Part model, mm, in its own coordinate system. Give positions to 0.01 mm unless a question says otherwise; leave off trailing zeros. Write each loop counter-clockwise with the first axis right and the second up, starting at its lowest first coordinate (ties: lowest second). Pieces come first, ordered by that corner, then holes. Notation, with made-up numbers: M 55,14 L 75,14 A16 ccw 75,33 Z; hole C 79.5,88.5 d3. An arc over 180 degrees is marked long. Use CSV: the item, a comma, the result in double quotes. Start each with the question number.
1. Band-saw the part on D-D, the plane x = 22.5. List the corners of the cut face in (y, z).
2. Drill centre lines: line 1 along X through (y, z) = (2.5, 0); line 2 along Z through (x, y) = (1, 2.4); line 3 along X through (y, z) = (1.2, -1). Where is each one in solid material? Low to high. Write a range as from..to.
3. Drop flat-ended pins along their axis: pin 1 Ø1 at (x, y) = (12, 2.5) entering from -Z; pin 2 Ø1 at (x, y) = (-5, 1.5) entering from -Z. Give the stop position or say it passes through.
4. Band-saw the part on A-A, the plane z = -81. List the corners of the cut face in (x, y), then the cut area to 3 significant figures.
5. Band-saw the part on B-B, the plane y = 2.05. Count the separate pieces of the cut face and the enclosed holes in it, then the cut area to 3 significant figures.
6. Band-saw the part on C-C, the plane z = -70. List the corners of the cut face in (x, y), then the cut area to 3 significant figures.
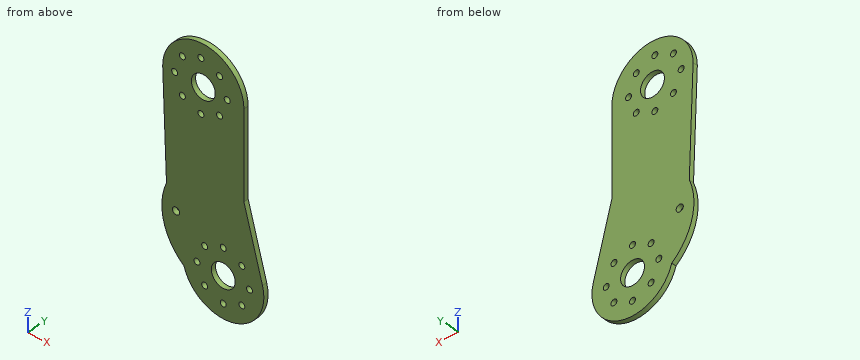
from build123d import *

# Parameters (mm, degrees)
RESSALTO_EXTRUS_O1_DEPTH      = 3
CORTE_EXTRUS_O8_REACH         = 92.666
ESBO_O7_R                     = 1.25
CORTE_EXTRUS_O9_REACH         = 92.666
ESBO_O8_R                     = 5
ESBO_O8_R_2                   = 1.5
CORTE_EXTRUS_O11_REACH        = 92.666
ESBO_O9_R                     = 1.25
CORTE_EXTRUS_O12_REACH        = 92.666
ESBO_O11_R                    = 5
CONVERTER_S_LIDO1_OUTLINE_R   = 1.25
CONVERTER_S_LIDO1_OUTLINE_R_2 = 5
CONVERTER_S_LIDO1_OUTLINE_R_3 = 1.5
CONVERTER_S_LIDO1_DEPTH       = 1


# Read off the part's stored shape, not the designer's step: Converter-Sólido1
with BuildPart() as part:
    # Esboço1 → Ressalto-extrusão1 (new body)
    with BuildSketch(Plane(origin=(0, 0, 0), x_dir=(1, 0, 0), z_dir=(0, 1, 0))):
        with BuildLine():
            Line((17, 36.622301445), (24.764571353, 65.600076233))
            ThreePointArc((24.764571353, 65.600076233), (12.765450327, 86.414910724), (-8.065221434, 74.443304555))
            ThreePointArc((-8.065221434, 74.443304555), (-16.588225274, 61.125706966), (-15.416069793, 45.357826591))
            Line((-15.416069793, 45.357826591), (-17, 0))
            ThreePointArc((-17, 0), (0, -17), (17, 0))
            Line((17, 0), (17, 36.622301445))
        make_face()
    extrude(amount=RESSALTO_EXTRUS_O1_DEPTH)

    # Esboço7 → Corte-extrusão8 (cut, up to next)
    with BuildSketch(Plane.XZ, mode=Mode.PRIVATE) as corte_extrus_o8_sk1:
        with Locations(Location((-1, -11, 0), (0, 0, 270))):
            Circle(ESBO_O7_R)
    corte_extrus_o8_tool1 = extrude(corte_extrus_o8_sk1.sketch, amount=-CORTE_EXTRUS_O8_REACH, mode=Mode.PRIVATE) & part.part
    # Esboço7 → Corte-extrusão8 (cut, up to next)
    with BuildSketch(Plane.XZ, mode=Mode.PRIVATE) as corte_extrus_o8_sk2:
        with Locations(Location((-8.778174593, -7.778174593, 0), (0, 0, 270))):
            Circle(ESBO_O7_R)
    corte_extrus_o8_tool2 = extrude(corte_extrus_o8_sk2.sketch, amount=-CORTE_EXTRUS_O8_REACH, mode=Mode.PRIVATE) & part.part
    # Esboço7 → Corte-extrusão8 (cut, up to next)
    with BuildSketch(Plane.XZ, mode=Mode.PRIVATE) as corte_extrus_o8_sk3:
        with Locations(Location((-12, 0, 0), (0, 0, 270))):
            Circle(ESBO_O7_R)
    corte_extrus_o8_tool3 = extrude(corte_extrus_o8_sk3.sketch, amount=-CORTE_EXTRUS_O8_REACH, mode=Mode.PRIVATE) & part.part
    # Esboço7 → Corte-extrusão8 (cut, up to next)
    with BuildSketch(Plane.XZ, mode=Mode.PRIVATE) as corte_extrus_o8_sk4:
        with Locations(Location((-8.778174593, 7.778174593, 0), (0, 0, 270))):
            Circle(ESBO_O7_R)
    corte_extrus_o8_tool4 = extrude(corte_extrus_o8_sk4.sketch, amount=-CORTE_EXTRUS_O8_REACH, mode=Mode.PRIVATE) & part.part
    # Esboço7 → Corte-extrusão8 (cut, up to next)
    with BuildSketch(Plane.XZ, mode=Mode.PRIVATE) as corte_extrus_o8_sk5:
        with Locations(Location((-1, 11, 0), (0, 0, 270))):
            Circle(ESBO_O7_R)
    corte_extrus_o8_tool5 = extrude(corte_extrus_o8_sk5.sketch, amount=-CORTE_EXTRUS_O8_REACH, mode=Mode.PRIVATE) & part.part
    # Esboço7 → Corte-extrusão8 (cut, up to next)
    with BuildSketch(Plane.XZ, mode=Mode.PRIVATE) as corte_extrus_o8_sk6:
        with Locations(Location((6.778174593, 7.778174593, 0), (0, 0, 270))):
            Circle(ESBO_O7_R)
    corte_extrus_o8_tool6 = extrude(corte_extrus_o8_sk6.sketch, amount=-CORTE_EXTRUS_O8_REACH, mode=Mode.PRIVATE) & part.part
    # Esboço7 → Corte-extrusão8 (cut, up to next)
    with BuildSketch(Plane.XZ, mode=Mode.PRIVATE) as corte_extrus_o8_sk7:
        with Locations(Location((10, 0, 0), (0, 0, 270))):
            Circle(ESBO_O7_R)
    corte_extrus_o8_tool7 = extrude(corte_extrus_o8_sk7.sketch, amount=-CORTE_EXTRUS_O8_REACH, mode=Mode.PRIVATE) & part.part
    # Esboço7 → Corte-extrusão8 (cut, up to next)
    with BuildSketch(Plane.XZ, mode=Mode.PRIVATE) as corte_extrus_o8_sk8:
        with Locations(Location((6.778174593, -7.778174593, 0), (0, 0, 270))):
            Circle(ESBO_O7_R)
    corte_extrus_o8_tool8 = extrude(corte_extrus_o8_sk8.sketch, amount=-CORTE_EXTRUS_O8_REACH, mode=Mode.PRIVATE) & part.part
    add(corte_extrus_o8_tool1.solids().sort_by_distance((-1, 0, -11))[0], mode=Mode.SUBTRACT)
    add(corte_extrus_o8_tool2.solids().sort_by_distance((-8.778175, 0, -7.778175))[0], mode=Mode.SUBTRACT)
    add(corte_extrus_o8_tool3.solids().sort_by_distance((-12, 0, 0))[0], mode=Mode.SUBTRACT)
    add(corte_extrus_o8_tool4.solids().sort_by_distance((-8.778175, 0, 7.778175))[0], mode=Mode.SUBTRACT)
    add(corte_extrus_o8_tool5.solids().sort_by_distance((-1, 0, 11))[0], mode=Mode.SUBTRACT)
    add(corte_extrus_o8_tool6.solids().sort_by_distance((6.778175, 0, 7.778175))[0], mode=Mode.SUBTRACT)
    add(corte_extrus_o8_tool7.solids().sort_by_distance((10, 0, 0))[0], mode=Mode.SUBTRACT)
    add(corte_extrus_o8_tool8.solids().sort_by_distance((6.778175, 0, -7.778175))[0], mode=Mode.SUBTRACT)

    # Esboço8 → Corte-extrusão9 (cut, up to next)
    with BuildSketch(Plane(origin=(0, 3, 0), x_dir=(1, 0, 0), z_dir=(0, 1, 0)), mode=Mode.PRIVATE) as corte_extrus_o9_sk1:
        with Locations(Location((0, 0, 0), (0, 0, 270))):
            Circle(ESBO_O8_R)
    corte_extrus_o9_tool1 = extrude(corte_extrus_o9_sk1.sketch, amount=-CORTE_EXTRUS_O9_REACH, mode=Mode.PRIVATE) & part.part
    # Esboço8 → Corte-extrusão9 (cut, up to next)
    with BuildSketch(Plane(origin=(0, 3, 0), x_dir=(1, 0, 0), z_dir=(0, 1, 0)), mode=Mode.PRIVATE) as corte_extrus_o9_sk2:
        with Locations(Location((-11.416069793, 54.443304555, 0), (0, 0, 270))):
            Circle(ESBO_O8_R_2)
    corte_extrus_o9_tool2 = extrude(corte_extrus_o9_sk2.sketch, amount=-CORTE_EXTRUS_O9_REACH, mode=Mode.PRIVATE) & part.part
    add(corte_extrus_o9_tool1.solids().sort_by_distance((0, 3, 0))[0], mode=Mode.SUBTRACT)
    add(corte_extrus_o9_tool2.solids().sort_by_distance((-11.41607, 3, -54.443305))[0], mode=Mode.SUBTRACT)

    # Esboço9 → Corte-extrusão11 (cut, up to next)
    with BuildSketch(Plane(origin=(0, 3, 0), x_dir=(1, 0, 0), z_dir=(0, 1, 0)), mode=Mode.PRIVATE) as corte_extrus_o11_sk1:
        with Locations(Location((8.343832306, 81, 0), (0, 0, 270))):
            Circle(ESBO_O9_R)
    corte_extrus_o11_tool1 = extrude(corte_extrus_o11_sk1.sketch, amount=-CORTE_EXTRUS_O11_REACH, mode=Mode.PRIVATE) & part.part
    # Esboço9 → Corte-extrusão11 (cut, up to next)
    with BuildSketch(Plane(origin=(0, 3, 0), x_dir=(1, 0, 0), z_dir=(0, 1, 0)), mode=Mode.PRIVATE) as corte_extrus_o11_sk2:
        with Locations(Location((16.122006899, 77.778174593, 0), (0, 0, 270))):
            Circle(ESBO_O9_R)
    corte_extrus_o11_tool2 = extrude(corte_extrus_o11_sk2.sketch, amount=-CORTE_EXTRUS_O11_REACH, mode=Mode.PRIVATE) & part.part
    # Esboço9 → Corte-extrusão11 (cut, up to next)
    with BuildSketch(Plane(origin=(0, 3, 0), x_dir=(1, 0, 0), z_dir=(0, 1, 0)), mode=Mode.PRIVATE) as corte_extrus_o11_sk3:
        with Locations(Location((19.343832306, 70, 0), (0, 0, 270))):
            Circle(ESBO_O9_R)
    corte_extrus_o11_tool3 = extrude(corte_extrus_o11_sk3.sketch, amount=-CORTE_EXTRUS_O11_REACH, mode=Mode.PRIVATE) & part.part
    # Esboço9 → Corte-extrusão11 (cut, up to next)
    with BuildSketch(Plane(origin=(0, 3, 0), x_dir=(1, 0, 0), z_dir=(0, 1, 0)), mode=Mode.PRIVATE) as corte_extrus_o11_sk4:
        with Locations(Location((16.122006899, 62.221825407, 0), (0, 0, 270))):
            Circle(ESBO_O9_R)
    corte_extrus_o11_tool4 = extrude(corte_extrus_o11_sk4.sketch, amount=-CORTE_EXTRUS_O11_REACH, mode=Mode.PRIVATE) & part.part
    # Esboço9 → Corte-extrusão11 (cut, up to next)
    with BuildSketch(Plane(origin=(0, 3, 0), x_dir=(1, 0, 0), z_dir=(0, 1, 0)), mode=Mode.PRIVATE) as corte_extrus_o11_sk5:
        with Locations(Location((8.343832306, 59, 0), (0, 0, 270))):
            Circle(ESBO_O9_R)
    corte_extrus_o11_tool5 = extrude(corte_extrus_o11_sk5.sketch, amount=-CORTE_EXTRUS_O11_REACH, mode=Mode.PRIVATE) & part.part
    # Esboço9 → Corte-extrusão11 (cut, up to next)
    with BuildSketch(Plane(origin=(0, 3, 0), x_dir=(1, 0, 0), z_dir=(0, 1, 0)), mode=Mode.PRIVATE) as corte_extrus_o11_sk6:
        with Locations(Location((0.565657713, 62.221825407, 0), (0, 0, 270))):
            Circle(ESBO_O9_R)
    corte_extrus_o11_tool6 = extrude(corte_extrus_o11_sk6.sketch, amount=-CORTE_EXTRUS_O11_REACH, mode=Mode.PRIVATE) & part.part
    # Esboço9 → Corte-extrusão11 (cut, up to next)
    with BuildSketch(Plane(origin=(0, 3, 0), x_dir=(1, 0, 0), z_dir=(0, 1, 0)), mode=Mode.PRIVATE) as corte_extrus_o11_sk7:
        with Locations(Location((-2.656167694, 70, 0), (0, 0, 270))):
            Circle(ESBO_O9_R)
    corte_extrus_o11_tool7 = extrude(corte_extrus_o11_sk7.sketch, amount=-CORTE_EXTRUS_O11_REACH, mode=Mode.PRIVATE) & part.part
    # Esboço9 → Corte-extrusão11 (cut, up to next)
    with BuildSketch(Plane(origin=(0, 3, 0), x_dir=(1, 0, 0), z_dir=(0, 1, 0)), mode=Mode.PRIVATE) as corte_extrus_o11_sk8:
        with Locations(Location((0.565657713, 77.778174593, 0), (0, 0, 270))):
            Circle(ESBO_O9_R)
    corte_extrus_o11_tool8 = extrude(corte_extrus_o11_sk8.sketch, amount=-CORTE_EXTRUS_O11_REACH, mode=Mode.PRIVATE) & part.part
    add(corte_extrus_o11_tool1.solids().sort_by_distance((8.343832, 3, -81))[0], mode=Mode.SUBTRACT)
    add(corte_extrus_o11_tool2.solids().sort_by_distance((16.122007, 3, -77.778175))[0], mode=Mode.SUBTRACT)
    add(corte_extrus_o11_tool3.solids().sort_by_distance((19.343832, 3, -70))[0], mode=Mode.SUBTRACT)
    add(corte_extrus_o11_tool4.solids().sort_by_distance((16.122007, 3, -62.221825))[0], mode=Mode.SUBTRACT)
    add(corte_extrus_o11_tool5.solids().sort_by_distance((8.343832, 3, -59))[0], mode=Mode.SUBTRACT)
    add(corte_extrus_o11_tool6.solids().sort_by_distance((0.565658, 3, -62.221825))[0], mode=Mode.SUBTRACT)
    add(corte_extrus_o11_tool7.solids().sort_by_distance((-2.656168, 3, -70))[0], mode=Mode.SUBTRACT)
    add(corte_extrus_o11_tool8.solids().sort_by_distance((0.565658, 3, -77.778175))[0], mode=Mode.SUBTRACT)

    # Esboço11 → Corte-extrusão12 (cut, up to next)
    with BuildSketch(Plane(origin=(0, 3, 0), x_dir=(1, 0, 0), z_dir=(0, 1, 0)), mode=Mode.PRIVATE) as corte_extrus_o12_sk1:
        with Locations(Location((8.343832306, 70, 0), (0, 0, 270))):
            Circle(ESBO_O11_R)
    corte_extrus_o12_tool1 = extrude(corte_extrus_o12_sk1.sketch, amount=-CORTE_EXTRUS_O12_REACH, mode=Mode.PRIVATE) & part.part
    add(corte_extrus_o12_tool1.solids().sort_by_distance((8.343832, 3, -70))[0], mode=Mode.SUBTRACT)

    # Converter-Sólido1 outline → Converter-Sólido1 (cut)
    with BuildSketch(Plane(origin=(0, 0, 0), x_dir=(1, 0, 0), z_dir=(0, 1, 0))):
        with BuildLine():
            ThreePointArc((24.764571353, 65.600076233), (12.765450327, 86.414910724), (-8.065221434, 74.443304555))
            ThreePointArc((-8.065221434, 74.443304555), (-16.588225274, 61.125706966), (-15.416069793, 45.357826591))
            Line((-15.416069793, 45.357826591), (-17, 0))
            ThreePointArc((-17, 0), (0, -17), (17, 0))
            Line((17, 0), (17, 36.622301445))
            Line((17, 36.622301445), (24.764571353, 65.600076233))
        make_face()
        with Locations((-8.778174593, -7.778174593)):
            Circle(CONVERTER_S_LIDO1_OUTLINE_R, mode=Mode.SUBTRACT)
        with Locations((-12, 0)):
            Circle(CONVERTER_S_LIDO1_OUTLINE_R, mode=Mode.SUBTRACT)
        with Locations((-8.778174593, 7.778174593)):
            Circle(CONVERTER_S_LIDO1_OUTLINE_R, mode=Mode.SUBTRACT)
        with Locations((-1, -11)):
            Circle(CONVERTER_S_LIDO1_OUTLINE_R, mode=Mode.SUBTRACT)
        Circle(CONVERTER_S_LIDO1_OUTLINE_R_2, mode=Mode.SUBTRACT)
        with Locations((-1, 11)):
            Circle(CONVERTER_S_LIDO1_OUTLINE_R, mode=Mode.SUBTRACT)
        with Locations((6.778174593, -7.778174593)):
            Circle(CONVERTER_S_LIDO1_OUTLINE_R, mode=Mode.SUBTRACT)
        with Locations((6.778174593, 7.778174593)):
            Circle(CONVERTER_S_LIDO1_OUTLINE_R, mode=Mode.SUBTRACT)
        with Locations((10, 0)):
            Circle(CONVERTER_S_LIDO1_OUTLINE_R, mode=Mode.SUBTRACT)
        with Locations((-11.416069793, 54.443304555)):
            Circle(CONVERTER_S_LIDO1_OUTLINE_R_3, mode=Mode.SUBTRACT)
        with Locations((-2.656167694, 70)):
            Circle(CONVERTER_S_LIDO1_OUTLINE_R, mode=Mode.SUBTRACT)
        with Locations((0.565657713, 62.221825407)):
            Circle(CONVERTER_S_LIDO1_OUTLINE_R, mode=Mode.SUBTRACT)
        with Locations((0.565657713, 77.778174593)):
            Circle(CONVERTER_S_LIDO1_OUTLINE_R, mode=Mode.SUBTRACT)
        with Locations((8.343832306, 59)):
            Circle(CONVERTER_S_LIDO1_OUTLINE_R, mode=Mode.SUBTRACT)
        with Locations((8.343832306, 70)):
            Circle(CONVERTER_S_LIDO1_OUTLINE_R_2, mode=Mode.SUBTRACT)
        with Locations((8.343832306, 81)):
            Circle(CONVERTER_S_LIDO1_OUTLINE_R, mode=Mode.SUBTRACT)
        with Locations((16.122006899, 62.221825407)):
            Circle(CONVERTER_S_LIDO1_OUTLINE_R, mode=Mode.SUBTRACT)
        with Locations((19.343832306, 70)):
            Circle(CONVERTER_S_LIDO1_OUTLINE_R, mode=Mode.SUBTRACT)
        with Locations((16.122006899, 77.778174593)):
            Circle(CONVERTER_S_LIDO1_OUTLINE_R, mode=Mode.SUBTRACT)
    extrude(amount=CONVERTER_S_LIDO1_DEPTH, mode=Mode.SUBTRACT)


solid = part.part
Output:
1,outline,"M 1,-79.41 L 3,-79.41 L 3,-57.15 L 1,-57.15 Z"
2,line 1,"x = -17..-13.25, -10.75..-5, 5..8.75, 11.25..17"
2,line 2,"z = -85.33..-78.95, -76.61..-63.39, -61.05..-4.9, 4.9..16.97"
2,line 3,"x = -16.97..-12.75, -11.25..-4.9, 4.9..9.25, 10.75..17"
3,pin 1,"stops at z = -86.7"
3,pin 2,"stops at z = -81.14"
4,outline,"M -4.62,1 L 7.09,1 L 7.09,3 L -4.62,3 Z; M 9.59,1 L 21.31,1 L 21.31,3 L 9.59,3 Z"
4,area,"46.8 mm²"
5,separate pieces,"1"
5,enclosed holes,"19"
5,area,"3,140 mm²"
6,outline,"M -12.35,1 L -3.91,1 L -3.91,3 L -12.35,3 Z; M -1.41,1 L 3.34,1 L 3.34,3 L -1.41,3 Z; M 13.34,1 L 18.09,1 L 18.09,3 L 13.34,3 Z; M 20.59,1 L 25.34,1 L 25.34,3 L 20.59,3 Z"
6,area,"45.4 mm²"
